Input: part model. Units: mm. Frame: model coordinates. Face numbers are marked on the shaded views. Give positions to 0.01 mm unless a question says otherwise; leave off trailing zeros. Loops run counter-clockwise (first coordinate to the right, second up) from the corner with the lowest first, then second, coordinate; pieces in that order, holes last. Notation, with made-up numbers: M 50,44.5 L 78,44.5 A20 cw 78,69.5 Z; hole C 47,88 d5. An arc over 180 degrees is marked long. Return JSON: item names as keys, results as strings. Group by question number.
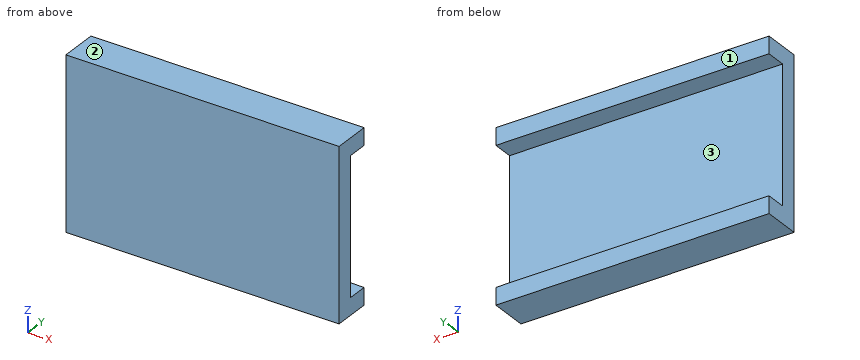
```python
from build123d import *

# Parameters (mm, degrees)
SKETCH1_W           = 80
SKETCH1_H           = 40
SKETCH1_H_2         = 5
BOSS_EXTRUDE2_DEPTH = 5
SKETCH2_W           = 80
SKETCH2_H           = 5
BOSS_EXTRUDE3_DEPTH = 6


with BuildPart() as part:
    # Sketch1 → Boss-Extrude2 (new body)
    with BuildSketch(Plane(origin=(0, 0, 0), x_dir=(1, 0, 0), z_dir=(0, 1, 0))):
        with Locations((40, 25)):
            Rectangle(SKETCH1_W, SKETCH1_H)
        with Locations((40, 2.5)):
            Rectangle(SKETCH1_W, SKETCH1_H_2)
        with Locations((40, 47.5)):
            Rectangle(SKETCH1_W, SKETCH1_H_2)
    extrude(amount=BOSS_EXTRUDE2_DEPTH)

    # Sketch2 → Boss-Extrude3 (add)
    with BuildSketch(Plane(origin=(0, 5, 0), x_dir=(1, 0, 0), z_dir=(0, 1, 0))):
        with Locations((40, 47.5)):
            Rectangle(SKETCH2_W, SKETCH2_H)
        with Locations((40, 2.5)):
            Rectangle(SKETCH2_W, SKETCH2_H)
    extrude(amount=BOSS_EXTRUDE3_DEPTH)


solid = part.part
```
Item 1: Section B-B, the plane x = 53.5. Return loops of the section in (y, z).
Item 2: Section C-C, the plane z = -36. Return loops of the section in (x, y).
Item 3: Section A-A, the plane y = 6.5. Return loops of the section in (x, z).
Item 4: Material intervals for line 1 (Z direction, x = 39, y = 10.5); line 2 (Y direction, x = 44, z = -23.5), sorted ascending. Write a range as from..to.
Item 5: Pull-direction query (Z, two-part tool) for the marked faces 1, 2 and 3; classes: pulls with the +Z half, pulls with the -Z half, needs draft (parallel to the pull), parting line crosses it, or undercut.
Item 6: First-contact query: pin 1 Ø1.8 at (x, y) = (46.5, 8.5) entering from +Z; pin 2 Ø2 at (y, z) = (7.5, -19.5) entering from -X; pin 3 Ø12 at (x, z) = (25, -34) entering from +Y. Flat tips, straight axial feed; report the tip coordinate or a pass-through.
Answer below:
{
 "1": {"outline": "M 0,-50 L 11,-50 L 11,-45 L 5,-45 L 5,-5 L 11,-5 L 11,0 L 0,0 Z"},
 "2": {"outline": "M 0,0 L 80,0 L 80,5 L 0,5 Z"},
 "3": {"outline": "M 0,-50 L 80,-50 L 80,-45 L 0,-45 Z; M 0,-5 L 80,-5 L 80,0 L 0,0 Z"},
 "4": {"line 1": "-50..-45, -5..0", "line 2": "0..5"},
 "5": {"face 1": "needs draft", "face 2": "pulls with the +Z half", "face 3": "undercut"},
 "6": {"pin 1": "z = 0", "pin 2": "through", "pin 3": "y = 5"}
}
